Could you check a few things on this model? Use its own coordinates, in mm. Give positions to 0.01 mm unless a question says otherwise; leave off trailing zeros. Order: outer loops, then holes, each group sorted by start corner. A loop starts at its lowest first (then second) coordinate and runs counter-clockwise, first axis right, second up. Notation, with made-up numbers: M -39.75,-2.75 L 10.25,-2.75 A16 ccw 10.25,13.25 Z; hole C -39.75,74.25 d9. An arc over 180 degrees is marked long. Use a Markdown table: item, result. Add a question column.
Item 1: Suppose I cut it at C-C on x = 20. Write out the boundary of the cut face in (y, z).
Item 2: I'm going to push flat-ended pins straight in: pin 1 Ø2.5 at (x, y) = (20, 30) entering from -Z; pin 2 Ø4 at (x, y) = (20, -30) entering from -Z. Where does each tip first touch, or does it pass through?
Item 3: If I drill on L1, parallel to Y at x = 20, z = 0.2; L2, parallel to Y at x = -20, z = 0.4; L3, parallel to Y at x = 21, z = 0.15, over which ranges is the centre line in solid material (lowest first)? Write a range as from..to.
Item 4: Suppose I cut it at B-B on x = -19.35. Write out the boundary of the cut face in (y, z) (3 decimals), plus the area to 3 significant figures.
Item 5: Suppose I cut it at A-A on y = 30. Write out the boundary of the cut face in (x, z), plus the area to 3 significant figures.
Autodesk Inventor part; units mm, degrees
ref_plane "YZ Plane" through (0, 0, 0) normal (1, 0, 0) x (0, 1, 0)
ref_plane "XZ Plane" through (0, 0, 0) normal (0, 1, 0) x (-1, 0, 0)
ref_plane "XY Plane" through (0, 0, 0) normal (0, 0, 1) x (1, 0, 0)
sketch "Sketch1" plane through (0, 0, 0) normal (0, 0, 1) x (1, 0, 0)
  line L0 (-25, 35) -> (25, 35)
  line L1 (25, 35) -> (25, -35)
  line L2 (25, -35) -> (-25, -35)
  line L3 (-25, -35) -> (-25, 35)
  line L4 (-25, 35) -> (25, -35) construction
  line L5 (25, 35) -> (-25, -35) construction
  circle A0 centre (-20, 30) radius 1.6
  line L6 (0, 0) -> (0, 8.6163)
  line L7 (0, 0) -> (6.049, 0)
  circle A1 centre (20, 30) radius 1.6
  circle A2 centre (-20, -30) radius 1.6
  circle A3 centre (20, -30) radius 1.6
  dimension "d0" = 50
  dimension "d1" = 70
  dimension "d12" = 3.2
  dimension "d13" = 5
  dimension "d18" = 5
extrude "Plate1" add sketch "Sketch1" along normal blind 1
sketch "Sketch2" plane through (0, 0, 1) normal (0, 0, 1) x (1, 0, 0)
  line L0 (22.55, 9.3405) -> (22.55, -9.3405)
  line L1 (22.55, -9.3405) -> (9.3405, -22.55)
  line L2 (9.3405, -22.55) -> (-9.3405, -22.55)
  line L3 (-9.3405, -22.55) -> (-22.55, -9.3405)
  line L4 (-22.55, -9.3405) -> (-22.55, 9.3405)
  line L5 (-22.55, 9.3405) -> (-9.3405, 22.55)
  line L6 (-9.3405, 22.55) -> (9.3405, 22.55)
  line L7 (9.3405, 22.55) -> (22.55, 9.3405)
  circle A0 centre (19.35, 8.015) radius 1.6
  line L8 (22.55, 9.3405) -> (-22.55, -9.3405)
  circle A1 centre (-19.35, -8.015) radius 1.6
  point P0 (0, 0)
  point P1 (0, 0)
  dimension "d3" = 45.1
  dimension "d4" = 3.2
  dimension "d5" = 3.2
  dimension "d8" = 360
extrude "Extrusion1" cut sketch "Sketch2" against normal blind 10 contours L8 A0 | A0 L8 | A1 L8 | L8 A1
equation "\"d2\" = 厚度"
equation "\"折彎半徑\" = 厚度"
equation "\"折彎離隙寬度\" = 厚度"
equation "\"折彎離隙深度\" = 0.5 * 厚度"
equation "\"轉角離隙大小\" = 4 * 厚度"
equation "\"最小剩餘\" = 2 * 厚度"
equation "\"轉移半徑\" = 折彎半徑"
equation "\"Jacobi半徑大小\" = 折彎半徑"
equation "\"間隙大小\" = 厚度"
properties part number "signal_combiner_plate" material "Aluminum"
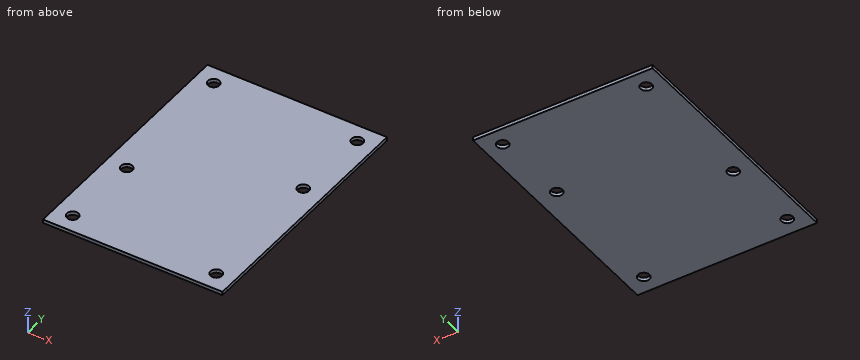
Findings below:
| question | item | result |
|---|---|---|
| 1 | outline | M -35,0 L -31.6,0 L -31.6,1 L -35,1 Z; M -28.4,0 L 6.55,0 L 6.55,1 L -28.4,1 Z; M 9.48,0 L 28.4,0 L 28.4,1 L 9.48,1 Z; M 31.6,0 L 35,0 L 35,1 L 31.6,1 Z |
| 2 | pin 1 | passes through |
| 2 | pin 2 | stops at z = 0 |
| 3 | L1 | y = -35..-31.6, -28.4..6.55, 9.48..28.4, 31.6..35 |
| 3 | L2 | y = -35..-31.6, -28.4..-9.48, -6.55..28.4, 31.6..35 |
| 3 | L3 | y = -35..-31.25, -28.75..28.75, 31.25..35 |
| 4 | outline | M -35,0 L -31.462,0 L -31.462,1 L -35,1 Z; M -28.538,0 L -9.615,0 L -9.615,1 L -28.538,1 Z; M -6.415,0 L 28.538,0 L 28.538,1 L -6.415,1 Z; M 31.462,0 L 35,0 L 35,1 L 31.462,1 Z |
| 4 | area | 61.0 mm^2 |
| 5 | outline | M -25,0 L -21.6,0 L -21.6,1 L -25,1 Z; M -18.4,0 L 18.4,0 L 18.4,1 L -18.4,1 Z; M 21.6,0 L 25,0 L 25,1 L 21.6,1 Z |
| 5 | area | 43.6 mm^2 |
